Could you check a few things on this model? Use its own coordinates, in mm. A direction names the side the tool comes from. Round coordinates to 2 decimals unless told otherwise and drop trailing zeros. Loops run counter-clockwise (first coordinate to the right, second up) from the corner with the lowest first, then second, coordinate; pieces in that order, holes last.
from build123d import *

# Parameters (mm, degrees)
SKETCH_1_R               = 8.475
EXTRUDE_1_DEPTH          = 24.1
CUT_EXTRUDE_2_REACH      = 28.916
SKETCH_3_R               = 5
EXTRUDE_2_DEPTH          = 22
SKETCH_6_R               = 12.5
SKETCH_6_R_2             = 7.5
EXTRUDE_3_DEPTH          = 3
EXTRUDE_START            = 1
SKETCH_20_R              = 8.8
SKETCH_20_R_2            = 8.475
EXTRUDE_4_DEPTH          = 1
HOLE_WIZARD_M3_4_D       = 2.5
HOLE_WIZARD_M3_4_DEPTH   = 8.5
HOLE_WIZARD_M3_4_TIP     = 0.751075774
SKETCH_24_R              = 30
EXTRUDE_5_DEPTH          = 5
SKETCH_25_R              = 2.5
CUT_EXTRUDE_3_DEPTH      = 10
HOLE_WIZARD_1_AT_2_COUNT = 2
HOLE_WIZARD_1_AT_2_PITCH = 22.5
HOLE_WIZARD_1_AT_3_COUNT = 2
HOLE_WIZARD_1_AT_3_PITCH = 38.97114317
HOLE_WIZARD_1_AT_4_COUNT = 2
HOLE_WIZARD_1_AT_4_PITCH = 45
HOLE_WIZARD_1_AT_5_COUNT = 2
HOLE_WIZARD_1_AT_5_PITCH = 38.97114317
HOLE_WIZARD_1_AT_6_COUNT = 2
HOLE_WIZARD_1_AT_6_PITCH = 22.5
EXTRUDE_START_2          = 4
SKETCH_34_R              = 8.475
SKETCH_34_R_2            = 5
EXTRUDE_8_DEPTH          = 4


with BuildPart() as part:
    # 草图1 → 凸台-拉伸1 (new body)
    with BuildSketch(Plane(origin=(0, 0, 0), x_dir=(1, 0, 0), z_dir=(0, 1, 0))):
        with Locations(Location((0, 0, 0), (0, 0, 270))):
            Circle(SKETCH_1_R)
    extrude(amount=EXTRUDE_1_DEPTH)

    # 草图3 → 切除-拉伸2 (cut, up to next)
    with BuildSketch(Plane.XZ, mode=Mode.PRIVATE) as cut_extrude_2_sk1:
        with Locations(Location((0, 0, 0), (0, 0, 270))):
            Circle(SKETCH_3_R)
    cut_extrude_2_tool1 = extrude(cut_extrude_2_sk1.sketch, amount=-CUT_EXTRUDE_2_REACH, mode=Mode.PRIVATE) & part.part
    add(cut_extrude_2_tool1.solids().sort_by_distance((0, 0, 0))[0], mode=Mode.SUBTRACT)

    # 草图4 → 凸台-拉伸2 (add)
    with BuildSketch(Plane.XZ):
        with BuildLine():
            Line((-3.947215931, 3.069118179), (-4.050917396, -2.930881821))
            ThreePointArc((-4.050917396, -2.930881821), (-4.999253362, 0.086404983), (-3.947215931, 3.069118179))
        make_face()
    extrude(amount=-EXTRUDE_2_DEPTH)

    # 草图6 → 凸台-拉伸3 (add)
    with BuildSketch(Plane(origin=(0, 24.1, 0), x_dir=(1, 0, 0), z_dir=(0, 1, 0))):
        with Locations(Location((0, 0, 0), (0, 0, 270))):
            Circle(SKETCH_6_R)
        Circle(SKETCH_6_R_2, mode=Mode.SUBTRACT)
    extrude(amount=-EXTRUDE_3_DEPTH)

    # 草图20 → 凸台-拉伸4 (add)
    with BuildSketch(Plane.XZ.offset(-21.1).offset(EXTRUDE_START)):
        with Locations(Location((0, 0, 0), (0, 0, 90))):
            Circle(SKETCH_20_R)
        with Locations(Location((0, 0, 0), (0, 0, 270))):
            Circle(SKETCH_20_R_2, mode=Mode.SUBTRACT)
    extrude(amount=-EXTRUDE_4_DEPTH)

    # M3 螺纹孔4
    with Locations(Plane(origin=(-3.999066663, 0, 0.069118179), x_dir=(-0.01728099666811417, 0, -0.9998506724277165), z_dir=(0.9998506724277165, 0, -0.01728099666811417))):
        with Locations((0, 10)):
            Hole(HOLE_WIZARD_M3_4_D / 2, depth=HOLE_WIZARD_M3_4_DEPTH)
            with Locations((0, 0, -(HOLE_WIZARD_M3_4_DEPTH + HOLE_WIZARD_M3_4_TIP / 2))):  # 118° drill point
                Cone(0, HOLE_WIZARD_M3_4_D / 2, HOLE_WIZARD_M3_4_TIP, mode=Mode.SUBTRACT)

    # 草图24 → 凸台-拉伸5 (add)
    with BuildSketch(Plane(origin=(0, 24.1, 0), x_dir=(1, 0, 0), z_dir=(0, 1, 0))):
        with Locations(Location((0, 0, 0), (0, 0, 270))):
            Circle(SKETCH_24_R)
    extrude(amount=EXTRUDE_5_DEPTH)

    # 草图25 → 切除-拉伸3 (cut)
    with BuildSketch(Plane(origin=(0, 29.1, 0), x_dir=(1, 0, 0), z_dir=(0, 1, 0))):
        with Locations(Location((0, 0, 0), (0, 0, 270))):
            Circle(SKETCH_25_R)
    extrude(amount=-CUT_EXTRUDE_3_DEPTH, mode=Mode.SUBTRACT)

    # 草图31 → 打孔尺寸(%根据十字)槽半沉头木螺钉的类型1 (revolve, cut)
    with BuildSketch(Plane(origin=(-11.275607113, 24.1, 19.47076486), x_dir=(0, 0, -1), z_dir=(1, 0, 0))):
        Polygon((0, 0), (0, 5), (2.75, 5), (2.75, 2.85), (5.6, 0), align=None)
    hole_wizard_1 = revolve(axis=Axis((-11.275607113, 17.75, 19.47076486), (0, 1, 0)), mode=Mode.SUBTRACT)

    # 打孔尺寸(%根据十字)槽半沉头木螺钉的类型1 at 2: 打孔尺寸(%根据十字)槽半沉头木螺钉的类型1 ×2
    with Locations(*[Vector(0.9999991358386731, 0, 0.0013146565738525046) * (i * HOLE_WIZARD_1_AT_2_PITCH) for i in range(1, HOLE_WIZARD_1_AT_2_COUNT)]):
        add(hole_wizard_1, mode=Mode.SUBTRACT)

    # 打孔尺寸(%根据十字)槽半沉头木螺钉的类型1 at 3: 打孔尺寸(%根据十字)槽半沉头木螺钉的类型1 ×2
    with Locations(*[Vector(0.8666819836857027, 0, -0.49886104192912833) * (i * HOLE_WIZARD_1_AT_3_PITCH) for i in range(1, HOLE_WIZARD_1_AT_3_COUNT)]):
        add(hole_wizard_1, mode=Mode.SUBTRACT)

    # 打孔尺寸(%根据十字)槽半沉头木螺钉的类型1 at 4: 打孔尺寸(%根据十字)槽半沉头木螺钉的类型1 ×2
    with Locations(*[Vector(0.5011380939095448, 0, -0.8653673271118504) * (i * HOLE_WIZARD_1_AT_4_PITCH) for i in range(1, HOLE_WIZARD_1_AT_4_COUNT)]):
        add(hole_wizard_1, mode=Mode.SUBTRACT)

    # 打孔尺寸(%根据十字)槽半沉头木螺钉的类型1 at 5: 打孔尺寸(%根据十字)槽半沉头木螺钉的类型1 ×2
    with Locations(*[Vector(0.0013146565738523764, 0, -0.9999991358386731) * (i * HOLE_WIZARD_1_AT_5_PITCH) for i in range(1, HOLE_WIZARD_1_AT_5_COUNT)]):
        add(hole_wizard_1, mode=Mode.SUBTRACT)

    # 打孔尺寸(%根据十字)槽半沉头木螺钉的类型1 at 6: 打孔尺寸(%根据十字)槽半沉头木螺钉的类型1 ×2
    with Locations(*[Vector(-0.49886104192912806, 0, -0.8666819836857028) * (i * HOLE_WIZARD_1_AT_6_PITCH) for i in range(1, HOLE_WIZARD_1_AT_6_COUNT)]):
        add(hole_wizard_1, mode=Mode.SUBTRACT)

    # 草图34 → 凸台-拉伸8 (add)
    with BuildSketch(Plane(origin=(0, 0, 0), x_dir=(-1, 0, 0), z_dir=(0, -1, 0)).offset(EXTRUDE_START_2)):
        with Locations(Location((0, 0, 0), (0, 0, 90))):
            Circle(SKETCH_34_R)
        with Locations(Location((0, 0, 0), (0, 0, 90))):
            Circle(SKETCH_34_R_2, mode=Mode.SUBTRACT)
    extrude(amount=-EXTRUDE_8_DEPTH)


solid = part.part
Item 1: If we section it at C-C, the plane z = 0: Count the separate pieces of the cut face and the enclosed holes in it, then the cut area to 3 significant figures.
Results list:
separate pieces: 5
enclosed holes: 0
area: 435 mm2
Item 2: We'd pull the mould along Z, two halves only. Please class faces 1 (the cylindrical face through (-8.725, 20.593, -1.146)), 2 (the conical face through (25.36, 26.77, 0.66)), 3 (the flat face through (-6, 29.1, 0)): released by +Z, released by -Z, zero draft, split by the parting line, or undercut.
Results list:
face 1: split by the parting line
face 2: undercut
face 3: zero draft
Item 3: For faces 4 (the flat face through (0, 24.1, 13)), 5 (the flat face through (-4, -4, -4)), which set-ups out of +Z, -Z, +X, -X, +Y, -Y let a thin tool reach every point of the face, with its end or its side?
Results list:
face 4: -Y
face 5: +Z, -Z, +X, -X, -Y
Item 4: If I drill on line 1 along X through (y, z) = (15.5, 0) (3 decimals); line 2 along Z through (x, y) = (9.5, 27); line 3 along Z through (x, y) = (0, -1.6) (3 decimals), over which ranges is the centre line in solid material (lowest first)?
Results list:
line 1: x = -8.475 to -4, 5 to 8.475
line 2: z = -28.46 to -21.57, -17.37 to 17.36, 21.64 to 28.46
line 3: z = -8.475 to -5, 5 to 8.475
Item 5: If we section it at A-A, the plane x = 0: Please give me the cut outline in (y, z) (3 decimals).
Results list:
outline: (-4, -8.475) - (20.1, -8.475) - (20.1, -8.8) - (21.1, -8.8) - (21.1, -12.5) - (24.1, -12.5) - (24.1, -30) - (29.1, -30) - (29.1, -2.5) - (24.1, -2.5) - (24.1, -5) - (-4, -5) - close; (-4, 5) - (24.1, 5) - (24.1, 2.5) - (29.1, 2.5) - (29.1, 30) - (24.1, 30) - (24.1, 12.5) - (21.1, 12.5) - (21.1, 8.8) - (20.1, 8.8) - (20.1, 8.475) - (-4, 8.475) - close
Item 6: If we section it at B-B, the plane y = 7: Please give me the cut outline in (x, z) (3 decimals).
Results list:
outline: circle Ø16.95 at (0, 0); hole (-4.051, -2.931) arc R5 ccw (long way) to (-3.947, 3.069) - close
Item 7: Will these pins go through, and if not, where does the flat tip stop? pin 1 (1.5 mm diameter, centred on y = 4, z = 1, fed in from +X); pin 2 (6.5 mm diameter, centred on x = 22.5, z = 0.03, fed in from -Y); pin 3 (9 mm diameter, centred on x = -11.22, z = -19.5, fed in from -Y); pin 4 (5 mm diameter, centred on x = -22.5, z = -0.03, fed in from -Y).
Results list:
pin 1: stops at x = 8.47
pin 2: stops at y = 26.45
pin 3: stops at y = 25.2
pin 4: passes through
